```python
from build123d import *

# Parameters (mm, degrees)
F0_W     = 60.5
F0_H     = 119
F0_R     = 3
F0_R_2   = 2.5
F0_R_3   = 1.5
F1_DEPTH = 3
F2_SIZE  = 1.5


with BuildPart() as f1:
    # F0 (on Top) → F1 (new body)
    with BuildSketch(Plane.XY):
        Rectangle(F0_W, F0_H)
        with Locations((-26.2, -55.4)):
            Circle(F0_R, mode=Mode.SUBTRACT)
        with Locations((26.2, -55.4)):
            Circle(F0_R, mode=Mode.SUBTRACT)
        with Locations((-26.2, 55.4)):
            Circle(F0_R, mode=Mode.SUBTRACT)
        with Locations((26.2, 55.4)):
            Circle(F0_R, mode=Mode.SUBTRACT)
        with BuildLine():
            Line((-8.082679, 69.293996), (-30.25, 59.5))
            Line((-30.25, 59.5), (30.25, 59.5))
            Line((30.25, 59.5), (8.082679, 69.293996))
            ThreePointArc((8.082679, 69.293996), (0, 71), (-8.082679, 69.293996))
        make_face()
        with Locations((0, 66.5)):
            Circle(F0_R_2, mode=Mode.SUBTRACT)
        with BuildLine():
            Line((30.25, -59.5), (-30.25, -59.5))
            Line((-30.25, -59.5), (-8.082679, -69.293996))
            ThreePointArc((-8.082679, -69.293996), (0, -71), (8.082679, -69.293996))
            Line((8.082679, -69.293996), (30.25, -59.5))
        make_face()
        with Locations((0, -66.5)):
            Circle(F0_R_2, mode=Mode.SUBTRACT)
        with Locations((-26.2, 55.4)):
            Circle(F0_R)
        with Locations((-26.2, 55.4)):
            Circle(F0_R_3, mode=Mode.SUBTRACT)
        with Locations((26.2, 55.4)):
            Circle(F0_R)
        with Locations((26.2, 55.4)):
            Circle(F0_R_3, mode=Mode.SUBTRACT)
        with Locations((-26.2, -55.4)):
            Circle(F0_R)
        with Locations((-26.2, -55.4)):
            Circle(F0_R_3, mode=Mode.SUBTRACT)
        with Locations((26.2, -55.4)):
            Circle(F0_R)
        with Locations((26.2, -55.4)):
            Circle(F0_R_3, mode=Mode.SUBTRACT)
    extrude(amount=F1_DEPTH)

    # F2
    f2_edges = [f1.edges().sort_by_distance(p)[0] for p in [
        (-27.7, 55.4, 3),
        (24.7, 55.4, 3),
        (24.7, -55.4, 3),
        (-27.7, -55.4, 3),
    ]]
    chamfer(f2_edges, length=F2_SIZE)


solid = f1.part
```
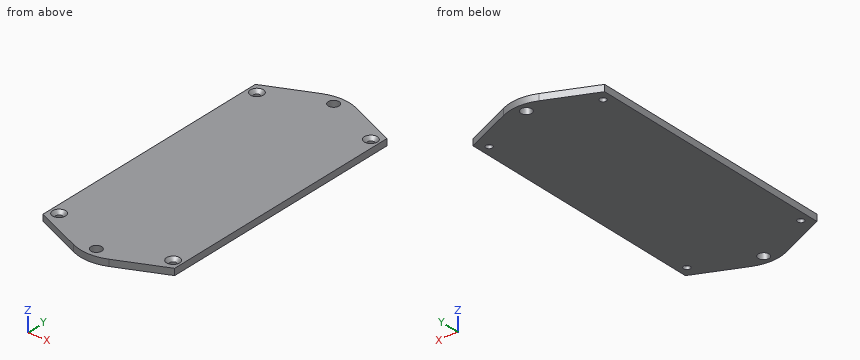
Verification items for the finished model (mm, model axes). Coordinates: 2 decimals unless noted, no trailing zeros. Write each loop counter-clockwise with the first axis right and the second up, starting at its lowest first coordinate (ties: lowest second). Pieces come first, ordered by that corner, then holes. Notation, with made-up numbers: M -26.5,-20 L 0.5,-20 A28 cw 0.5,1 Z; hole C 18,-19 d4. An arc over 180 degrees is marked long. Answer as a JSON object with one key per item and string values. Group by question number.
(1) Cross-section at C-C, the plane x = -26.2. Record the cut outline in (y, z), and give its area (3 significant figures).
(2) Gauge pin test, flat end, axial feed: pin 1 (1.8 mm diameter, centred on x = -26.2, y = 55.4, fed in from +Z). Record the tip position at first contact, or that the pin passes through.
(3) Cross-section at B-B, the plane z = 2. Record the cut outline in (x, y).
(4) Material ranges on line 1 (Y direction, x = 26.2, z = 0.85); line 2 (Y direction, x = 25, z = 1.55); line 3 (X direction, y = -53.5, z = 2.3), recorded low to high.
(5) Cross-section at A-A, the plane y = 55.4. Record the cut outline in (x, z).
(6) Cross-section at D-D, the plane x = 10. Record the cut outline in (y, z).
Reply:
{
 "1": {"outline": "M -61.29,0 L -56.9,0 L -56.9,1.5 L -58.4,3 L -61.29,3 Z; M -53.9,0 L 53.9,0 L 53.9,1.5 L 52.4,3 L -52.4,3 L -53.9,1.5 Z; M 56.9,0 L 61.29,0 L 61.29,3 L 58.4,3 L 56.9,1.5 Z", "area": "345 mm²"},
 "2": {"pin 1": "through"},
 "3": {"outline": "M -30.25,-59.5 L -8.08,-69.29 A20 ccw 8.08,-69.29 L 30.25,-59.5 L 30.25,59.5 L 8.08,69.29 A20 ccw -8.08,69.29 L -30.25,59.5 Z; hole C -26.2,-55.4 d4; hole C -26.2,55.4 d4; hole C 0,-66.5 d5; hole C 0,66.5 d5; hole C 26.2,-55.4 d4; hole C 26.2,55.4 d4"},
 "4": {"line 1": "-61.29 to -56.9, -53.9 to 53.9, 56.9 to 61.29", "line 2": "-61.82 to -56.38, -54.42 to 54.42, 56.38 to 61.82", "line 3": "-30.25 to -27.5, -24.9 to 24.9, 27.5 to 30.25"},
 "5": {"outline": "M -30.25,0 L -27.7,0 L -27.7,1.5 L -29.2,3 L -30.25,3 Z; M -24.7,0 L 24.7,0 L 24.7,1.5 L 23.2,3 L -23.2,3 L -24.7,1.5 Z; M 27.7,0 L 30.25,0 L 30.25,3 L 29.2,3 L 27.7,1.5 Z"},
 "6": {"outline": "M -68.45,0 L 68.45,0 L 68.45,3 L -68.45,3 Z"}
}
